Geometry: final body of the model. Coordinates: model frame, mm. Give positions to 0.01 mm unless a question says otherwise; leave off trailing zeros. Order: outer loops, then holes, each group sorted by start corner. A loop starts at its lowest first (then second) coordinate and runs counter-clockwise, first axis right, second up. Notation, with made-up numbers: (35.25, 7) - (69.25, 7) arc R24 ccw to (69.25, 29) - close; hole circle Ø1 at (-29, -17). An arc over 180 degrees is marked (long way). One line per question, with ' | ' between items. Start each with the question number.
from build123d import *

# Parameters (mm, degrees)
SKETCH_1_R      = 35.5
SKETCH_1_R_2    = 2.25
EXTRUDE_1_DEPTH = 5


with BuildPart() as part:
    # Эскиз1 → Бобышка-Вытянуть1 (new body)
    with BuildSketch(Plane(origin=(0, 0, 0), x_dir=(1, 0, 0), z_dir=(0, 1, 0))):
        with BuildLine():
            Line((-47.236109069, -55), (47.236109069, -55))
            ThreePointArc((47.236109069, -55), (72.5, 0), (47.236109069, 55))
            Line((47.236109069, 55), (-47.236109069, 55))
            ThreePointArc((-47.236109069, 55), (-72.5, 0), (-47.236109069, -55))
        make_face()
        Circle(SKETCH_1_R, mode=Mode.SUBTRACT)
        with Locations((53.220649991, 27.704916794)):
            Circle(SKETCH_1_R_2, mode=Mode.SUBTRACT)
        with Locations((53.220649991, -27.704916794)):
            Circle(SKETCH_1_R_2, mode=Mode.SUBTRACT)
        with Locations((-53.220649991, -27.704916794)):
            Circle(SKETCH_1_R_2, mode=Mode.SUBTRACT)
        with Locations((-53.220649991, 27.704916794)):
            Circle(SKETCH_1_R_2, mode=Mode.SUBTRACT)
    extrude(amount=EXTRUDE_1_DEPTH)


solid = part.part
(1) Material intervals for line 1 along Z through (x, y) = (0, 2); line 2 along Z through (x, y) = (52, 1.5); line 3 along X through (y, z) = (1.75, -2.5), sorted ascending. Write a range as from..to.
(2) Cut plane C-C, the plane x = 0. Return the cut outline in (y, z), plus the area to 3 significant figures.
(3) Cut plane A-A, the plane z = 0. Return the cut outline in (x, y), plus the area to 3 significant figures.
(4) Cut plane D-D, the plane y = 3.85. Return the cut outline in (x, z).
(5) Cut plane B-B, the plane x = 53. Return the cut outline in (y, z).
(6) Pull-direction query (X, two-part tool) for faces 1 (the cylindrical face through (50.973, 2.465, 27.606)), 2 (the cylindrical face through (-72.495, 2.465, -0.874)), 3 (the flat face through (1, 2, -55)); classes: +X half, -X half, draft (parallel to the pull), parting line (faces both ways), or undercut.
(7) Contact query for a flat-ended pin moving along its axis: P1, Ø2.5, axis at x = -53.22, z = 27.7, coming from the +Y side. Output: stop coordinate, or through.
Results are:
1) line 1: -55..-35.5, 35.5..55 | line 2: -50.52..-29.6, -25.81..25.81, 29.6..50.52 | line 3: -72.46..-35.41, 35.41..72.46
2) outline: (0, -55) - (5, -55) - (5, -35.5) - (0, -35.5) - close; (0, 35.5) - (5, 35.5) - (5, 55) - (0, 55) - close | area: 195 mm2
3) outline: (-72.5, 0) - (-35.5, 0) - (-35.5, 5) - (-72.5, 5) - close; (35.5, 0) - (72.5, 0) - (72.5, 5) - (35.5, 5) - close | area: 370 mm2
4) outline: (-47.24, -55) - (47.24, -55) arc R72.5 ccw to (47.24, 55) - (-47.24, 55) arc R72.5 ccw to start; hole circle Ø4.5 at (-53.22, -27.7); hole circle Ø4.5 at (-53.22, 27.7); hole circle Ø71 at (0, 0); hole circle Ø4.5 at (53.22, -27.7); hole circle Ø4.5 at (53.22, 27.7)
5) outline: (0, -49.47) - (5, -49.47) - (5, -29.94) - (0, -29.94) - close; (0, -25.47) - (5, -25.47) - (5, 25.47) - (0, 25.47) - close; (0, 29.94) - (5, 29.94) - (5, 49.47) - (0, 49.47) - close
6) face 1: undercut | face 2: -X half | face 3: draft
7) P1: through
